Build history of the part. All positions in model axes, mm. A direction names the side the tool comes from. Give positions to 0.01 mm unless a question says otherwise; leave off trailing zeros. Write each loop counter-clockwise with the first axis right and the second up, starting at its lowest first coordinate (ties: lowest second). Pieces come first, ordered by that corner, then holes. Notation, with made-up numbers: (-7, 52.5) -> (6, 52.5) arc R10 cw to (6, 63.5) -> close; hole circle Ø5 at (-8.75, 32). An arc over 180 degrees is marked (long way). Write item = value, one per line. Start each with the question number.
Q1. Wall check: line 1 (Y direction, x = 15.5, z = 18.5); line 2 (Y direction, x = 16.5, z = 19.75); line 3 (Y direction, x = 17, z = 19). Give the ranges that are in metal, low to high.
Q2. Saw through at B-B, the plane x = 19. List the corners of the cut face in (y, z).
Q3. Saw through at A-A, the plane x = 15.5. List the corners of the cut face in (y, z), then the cut area to 3 significant figures.
Q4. Drop flat-ended pins along their axis: P1, Ø1.5, axis at x = 14, y = 33.5, coming from the +Z side; P2, Ø2.5, axis at y = 44, z = 23.5, coming from the -X side. Give the stop position or say it passes through.
Q5. Tool access for faces 1 (the face through (18.22, 48.619, 21.585)), 2 (the face through (11, 37, 23)): list every direction of +Z, -Z, +X, -X, +Y, -Y with a clear straight run to the whole face (end or side of a thin tool).
from build123d import *

# Parameters (mm, degrees)
SKETCH152_W      = 9
SKETCH152_H      = 35
SKETCH152_R      = 2.1
PAD086_DEPTH     = 20
CHAMFER056_SIZE  = 2
HOLE_D           = 3.2
HOLE_CBORE_D     = 10
HOLE_CBORE_DEPTH = 3.2
CHAMFER057_SIZE  = 0.4
CHAMFER058_SIZE  = 2.5
CHAMFER059_SIZE  = 0.4


with BuildPart() as part:
    # Sketch152 → Pad086 (new body)
    with BuildSketch(Plane.XY):
        with Locations((0, 8.5)):
            Rectangle(SKETCH152_W, SKETCH152_H)
        with Locations((0, 4)):
            Circle(SKETCH152_R, mode=Mode.SUBTRACT)
        with Locations((0, -4)):
            Circle(SKETCH152_R, mode=Mode.SUBTRACT)
    extrude(amount=PAD086_DEPTH)

    # Chamfer056
    chamfer056_edges = [part.edges().sort_by_distance(p)[0] for p in [
        (4.5, -9, 10),
        (-4.5, -9, 10),
        (-4.5, 26, 10),
        (4.5, 26, 10),
    ]]
    chamfer(chamfer056_edges, length=CHAMFER056_SIZE)

    # Hole (through all)
    with Locations(Plane.YZ.offset(4.5)):
        with Locations((15, 10)):
            CounterBoreHole(HOLE_D / 2, HOLE_CBORE_D / 2, HOLE_CBORE_DEPTH)

    # Chamfer057
    chamfer057_edges = [part.edges().sort_by_distance(p)[0] for p in [
        (1.3, 15, 11.6),
        (4.5, 15, 15),
    ]]
    chamfer(chamfer057_edges, length=CHAMFER057_SIZE)

    # Chamfer058
    chamfer058_edges = [part.edges().sort_by_distance(p)[0] for p in [
        (-4.5, 15, 11.6),
    ]]
    chamfer(chamfer058_edges, length=CHAMFER058_SIZE)

    # Chamfer059
    chamfer059_edges = [part.edges().sort_by_distance(p)[0] for p in [
        (-2.1, 4, 20),
        (-2.1, -4, 20),
        (-2.1, 4, 0),
        (-2.1, -4, 0),
    ]]
    chamfer(chamfer059_edges, length=CHAMFER059_SIZE)


with BuildPart() as part_1:
    # Body074 placement: moved
    add(part.part.moved(Location((15.5, 28.999977, 13.499984))))


solid = part_1.part
Report:
q1.line_1 = 20 to 22.9, 27.1 to 30.9, 35.1 to 55
q1.line_2 = 20 to 23.15, 26.85 to 31.15, 34.85 to 55
q1.line_3 = 20 to 23.53, 26.47 to 31.53, 34.47 to 41.82, 46.18 to 55
q2.outline = (21, 13.5) -> (54, 13.5) -> (54, 33.5) -> (21, 33.5) -> close; hole circle Ø10 at (44, 23.5)
q3.outline = (20, 13.5) -> (22.5, 13.5) -> (22.9, 13.9) -> (22.9, 33.1) -> (22.5, 33.5) -> (20, 33.5) -> close; (27.1, 13.9) -> (27.5, 13.5) -> (30.5, 13.5) -> (30.9, 13.9) -> (30.9, 33.1) -> (30.5, 33.5) -> (27.5, 33.5) -> (27.1, 33.1) -> close; (35.1, 13.9) -> (35.5, 13.5) -> (55, 13.5) -> (55, 33.5) -> (35.5, 33.5) -> (35.1, 33.1) -> close; hole circle Ø3.2 at (44, 23.5)
q3.area = 523 mm2
q4.P1 = 33.33
q4.P2 = through
q5.face_1 = +X
q5.face_2 = +Z, -Z, -X, +Y, -Y
